from build123d import *

# Parameters (mm, degrees)
EXTRUDE_1_DEPTH          = 1000
EXTRUDE_2_DEPTH          = 100
CUT_EXTRUDE_3_DEPTH      = 20
CUT_EXTRUDE_3_DEPTH_BACK = 842.888353643


with BuildPart() as part:
    # Эскиз2 → Бобышка-Вытянуть1 (new body)
    with BuildSketch(Plane.XY):
        Polygon((0, 0), (-10, 0), (-10, 20), (-20, 20), (-20, -10), (0, -10), (20, -10), (20, 20), (10, 20), (10, 0), align=None)
    extrude(amount=EXTRUDE_1_DEPTH)

    # Эскиз5 → Бобышка-Вытянуть2 (add)
    with BuildSketch(Plane.XY.offset(100)):
        with BuildLine():
            Line((-20, 20), (-10, 20))
            ThreePointArc((-10, 20), (0, 21.622776602), (10, 20))
            Line((10, 20), (20, 20))
            ThreePointArc((20, 20), (0, 26.055512755), (-20, 20))
        make_face()
    extrude(amount=EXTRUDE_2_DEPTH)

    # Sketch 5 2 → Вырез-Вытянуть3 (cut, two sides: drawn at the far end of the back side and taken through both)
    with BuildSketch(Plane(origin=(30, 16, 160), x_dir=(0, 0.1961161351381843, -0.9805806756909201), z_dir=(-1, 0, 0)).offset(-CUT_EXTRUDE_3_DEPTH_BACK)):
        Polygon((0, 0), (0.784464541, -3.922322703), (20.396078054, 0), (19.611613514, 3.922322703), align=None)
    extrude(amount=CUT_EXTRUDE_3_DEPTH + CUT_EXTRUDE_3_DEPTH_BACK, mode=Mode.SUBTRACT)


solid = part.part
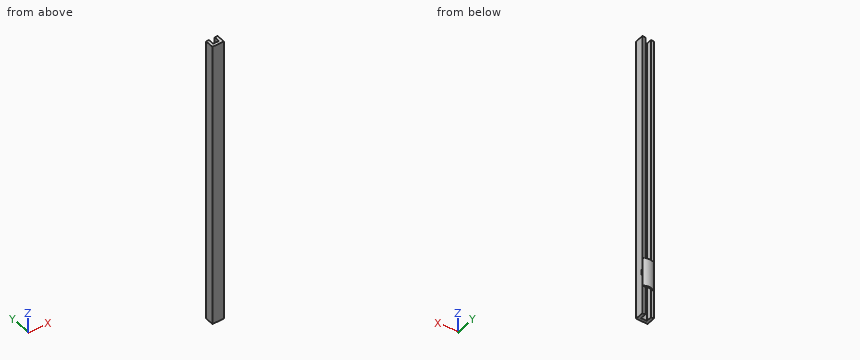
Can you work these out from the model? Positions are in its coordinate system, mm. Round coordinates to 2 decimals unless told otherwise and drop trailing zeros. Order: outer loops, then holes, each group sorted by start corner. A loop starts at its lowest first (then second) coordinate and runs counter-clockwise, first axis right, second up. Notation, with made-up numbers: (68, 29) - (96, 29) arc R14 ccw to (96, 45) - close; hole circle Ø2 at (-18, -38). An arc over 180 degrees is marked (long way). Answer in a Markdown table with one row per item.
(1) Suppose I cut it at A-A, the plane y = 9. Please give me the cut outline in (x, z), plus the area to 3 significant figures.
From the geometry:
| item | result |
|---|---|
| outline | (-20, 0) - (-10, 0) - (-10, 1000) - (-20, 1000) - close; (10, 0) - (20, 0) - (20, 1000) - (10, 1000) - close |
| area | 20,000 mm2 |
(2) Suppose I cut it at B-B, the plane x = 2. Please give me the cut outline in (y, z), plus the area to 3 significant figures.
From the geometry:
| item | result |
|---|---|
| outline | (-10, 0) - (0, 0) - (0, 1000) - (-10, 1000) - close; (21.56, 100) - (26, 100) - (26, 200) - (21.56, 200) - close |
| area | 10,400 mm2 |
(3) For P1, Ø10, axis at x = 1.5, z = 402, coming from the +Y side; P2, Ø5, axis at x = -17.5, z = 678, coming from the +Y side; P3, Ø1.8, axis at x = -7, y = 23.5, coming from the +Z side; P4, Ø4, axis at x = -6.5, y = -1, coming from the -Z side, each with a flat end and sliding along its axis, tell me the tip position at first contact or that it passes through.
From the geometry:
| item | result |
|---|---|
| P1 | stops at y = 0 |
| P2 | stops at y = 20 |
| P3 | stops at z = 200 |
| P4 | stops at z = 0 |
(4) Please list where these lines run through material, in increasing order: L1, parallel to X at y = 2.5, z = 737.5; L2, parallel to Y at x = -18, z = 77; L3, parallel to Y at x = -3, z = 486.5. Write a range as from..to.
From the geometry:
| item | result |
|---|---|
| L1 | x = -20..-10, 10..20 |
| L2 | y = -10..20 |
| L3 | y = -10..0 |
(5) Suppose I cut it at C-C, the plane z = 842. Please give me the cut outline in (x, y).
From the geometry:
| item | result |
|---|---|
| outline | (-20, -10) - (20, -10) - (20, 20) - (10, 20) - (10, 0) - (-10, 0) - (-10, 20) - (-20, 20) - close |
